Input: part model. Units: mm. Frame: model coordinates. A direction names the side the tool comes from. Round coordinates to 2 decimals unless told otherwise and drop trailing zeros. Loops run counter-clockwise (first coordinate to the right, second up) from the corner with the lowest first, then second, coordinate; pieces in that order, holes last. Notation, with made-up numbers: (-8, 37) -> (2, 37) arc R16 ccw to (2, 59) -> close; hole circle Ø1 at (44.25, -29). An arc over 180 degrees is marked (long way). Answer as a JSON object with one key per item and string values. Group by question number.
Item 1: Set-up query: faces 1 (the flat face through (22.225, -13, 54)), 2 (the flat face through (13, -22.225, 22)), 3 (the flat face through (3.175, -13, 54)), 4 (the cylindrical face through (21.5, -3.94, 54.02)), 5 (the flat face through (6.35, -13, 54)). Return all of +Z, -Z, +X, -X, +Y, -Y with unobstructed straight access to the full face (end or side cutting, diameter ignored); none if empty.
Item 2: Section query D-D on z = 42. Return loops of the section in (x, y) (3 decimals).
Item 3: Section query B-B on y = -16. Return loops of the section in (x, z) (3 decimals).
Item 4: Section query C-C on x = 13.75. Return loops of the section in (y, z) (3 decimals), and give its area (3 significant figures).
Item 5: Material intervals for line 1 (X direction, y = -21.75, z = 42.5) (3 decimals); line 2 (Y direction, x = 11, z = 14) (3 decimals); line 3 (Y direction, x = 18.5, z = 52) (3 decimals), sorted ascending. Write a range as [from, to].
Item 6: Section query A-A on z = 54. Return loops of the section in (x, y) (3 decimals), and give its area (3 significant figures).
Item 7: Draft query along Y for faces 6 (the cylindrical face through (3.94, -21.5, 54.02)), 7 (the cylindrical face through (3.94, -3.9, 54.02)), 8 (the flat face through (19.05, -13, 54)). Return one class per face: released by +Y, released by -Y, zero draft, split by the parting line, or undercut.
Item 8: Pin query (flat end, axial travel): pin 1 (5 mm diameter, centred on x = 14.5, z = 54, fed in from +Y) (3 decimals); pin 2 (3 mm diameter, centred on y = -14.5, z = 54, fed in from -X) (3 decimals); pin 3 (3 mm diameter, centred on y = -13.5, z = 52.5, fed in from +X) (3 decimals). Return the tip coordinate at first contact, or that it passes through.
from build123d import *

# Parameters (mm, degrees)
F0_W     = 25.4
F0_H     = 25.4
F1_DEPTH = 50.8
F2_W     = 19.05
F2_H     = 19.05
F3_DEPTH = 44.45
F4_W     = 19.05
F4_H     = 19.05
F4_W_2   = 12.7
F4_H_2   = 12.7
F5_DEPTH = 6.35
F6_R     = 2.54


# Not quite as in the source:
# - a feature names something its author has since deleted; it is built from what else it names


with BuildPart() as f1:
    # F0 (on Top) → F1 (new body)
    with BuildSketch(Plane.XY):
        with Locations((12.7, -12.7)):
            Rectangle(F0_W, F0_H)
    extrude(amount=F1_DEPTH)

    # F2 (on face) → F3 (cut)
    with BuildSketch(Plane(origin=(0, 0, 0), x_dir=(1, 0, 0), z_dir=(0, 0, -1))):
        with Locations((12.7, 12.7)):
            Rectangle(F2_W, F2_H)
    extrude(amount=-F3_DEPTH, mode=Mode.SUBTRACT)

    # F4 (on face) → F5 (join)
    with BuildSketch(Plane.XY.offset(50.8)):
        with Locations((12.7, -12.7)):
            Rectangle(F4_W, F4_H)
        with Locations((12.7, -12.7)):
            Rectangle(F4_W_2, F4_H_2, mode=Mode.SUBTRACT)
    extrude(amount=F5_DEPTH)

    # F6
    f6_edges = [f1.edges().sort_by_distance(p)[0] for p in [
        (0, 0, 25.4),
        (0, -25.4, 25.4),
        (25.4, 0, 25.4),
        (3.175, -3.175, 53.975),
        (3.175, -22.225, 53.975),
        (22.225, -3.175, 53.975),
        (22.225, -22.225, 53.975),
        (25.4, -25.4, 25.4),
    ]]
    fillet(f6_edges, radius=F6_R)


solid = f1.part
Solved:
{
 "1": {"face 1": "+Z, +X, +Y, -Y", "face 2": "-Z", "face 3": "+Z, -X, +Y, -Y", "face 4": "+Z, +X, +Y", "face 5": "+Z"},
 "2": {"outline": "(0, -22.86) arc R2.54 ccw to (2.54, -25.4) -> (22.86, -25.4) arc R2.54 ccw to (25.4, -22.86) -> (25.4, -2.54) arc R2.54 ccw to (22.86, 0) -> (2.54, 0) arc R2.54 ccw to (0, -2.54) -> close; hole (3.175, -22.225) -> (22.225, -22.225) -> (22.225, -3.175) -> (3.175, -3.175) -> close"},
 "3": {"outline": "(0, 0) -> (3.175, 0) -> (3.175, 44.45) -> (22.225, 44.45) -> (22.225, 0) -> (25.4, 0) -> (25.4, 50.8) -> (22.225, 50.8) -> (22.225, 57.15) -> (19.05, 57.15) -> (19.05, 50.8) -> (6.35, 50.8) -> (6.35, 57.15) -> (3.175, 57.15) -> (3.175, 50.8) -> (0, 50.8) -> close"},
 "4": {"outline": "(-25.4, 0) -> (-22.225, 0) -> (-22.225, 44.45) -> (-3.175, 44.45) -> (-3.175, 0) -> (0, 0) -> (0, 50.8) -> (-3.175, 50.8) -> (-3.175, 57.15) -> (-6.35, 57.15) -> (-6.35, 50.8) -> (-19.05, 50.8) -> (-19.05, 57.15) -> (-22.225, 57.15) -> (-22.225, 50.8) -> (-25.4, 50.8) -> close", "area": "484 mm²"},
 "5": {"line 1": "[0, 3.175], [22.225, 25.4]", "line 2": "[-25.4, -22.225], [-3.175, 0]", "line 3": "[-22.225, -19.05], [-6.35, -3.175]"},
 "6": {"outline": "(3.175, -19.685) arc R2.54 ccw to (5.715, -22.225) -> (19.685, -22.225) arc R2.54 ccw to (22.225, -19.685) -> (22.225, -5.715) arc R2.54 ccw to (19.685, -3.175) -> (5.715, -3.175) arc R2.54 ccw to (3.175, -5.715) -> close; hole (6.35, -19.05) -> (19.05, -19.05) -> (19.05, -6.35) -> (6.35, -6.35) -> close", "area": "196 mm²"},
 "7": {"face 6": "released by -Y", "face 7": "released by +Y", "face 8": "undercut"},
 "8": {"pin 1": "y = -3.175", "pin 2": "x = 3.175", "pin 3": "x = 22.225"}
}
